The listing builds one solid part. Answer for the finished solid, in the listing's coordinates (mm). A direction names the side the tool comes from. Give positions to 0.01 mm unless a question says otherwise; leave off trailing zeros. Order: outer loops, then holes, each group sorted by start corner. A loop starts at its lowest first (then second) coordinate and runs counter-clockwise, first axis right, second up. Notation, with made-up numbers: (62.5, 57) -> (121.5, 57) arc R15 cw to (121.5, 69) -> close; hole circle Ø4 at (-27.5, -25). An arc over 180 degrees is marked (long way). Answer as a JSON object with one key per item and string values. Group by question number.
```python
from build123d import *

# Parameters (mm, degrees)
SKETCH1_R           = 0.75
SKETCH1_R_2         = 0.5
BOSS_EXTRUDE1_DEPTH = 2


with BuildPart() as part:
    # Sketch1 → Boss-Extrude1 (new body)
    with BuildSketch(Plane.XY):
        with BuildLine():
            Line((3.1, 16.98), (-3.1, 16.98))
            ThreePointArc((-3.1, 16.98), (-6.635533906, 15.515533906), (-8.1, 11.98))
            Line((-8.1, 11.98), (-8.1, 6))
            Line((-8.1, 6), (-4.1, 6))
            Line((-4.1, 6), (-4.1, 4))
            Line((-4.1, 4), (-8.1, 4))
            Line((-8.1, 4), (-8.1, 2))
            ThreePointArc((-8.1, 2), (-7.514213562, 0.585786438), (-6.1, 0))
            Line((-6.1, 0), (6.1, 0))
            ThreePointArc((6.1, 0), (7.514213562, 0.585786438), (8.1, 2))
            Line((8.1, 2), (8.1, 4))
            Line((8.1, 4), (4.1, 4))
            Line((4.1, 4), (4.1, 6))
            Line((4.1, 6), (8.1, 6))
            Line((8.1, 6), (8.1, 11.98))
            ThreePointArc((8.1, 11.98), (6.635533906, 15.515533906), (3.1, 16.98))
        make_face()
        with Locations((-5.35, 2)):
            Circle(SKETCH1_R, mode=Mode.SUBTRACT)
        with Locations((-5.1, 13.98)):
            Circle(SKETCH1_R_2, mode=Mode.SUBTRACT)
        with Locations((-2.1, 8.5)):
            Circle(SKETCH1_R, mode=Mode.SUBTRACT)
        with Locations((2.1, 8.5)):
            Circle(SKETCH1_R, mode=Mode.SUBTRACT)
        with Locations((5.1, 13.98)):
            Circle(SKETCH1_R_2, mode=Mode.SUBTRACT)
        with Locations((5.35, 2)):
            Circle(SKETCH1_R, mode=Mode.SUBTRACT)
    extrude(amount=BOSS_EXTRUDE1_DEPTH)


solid = part.part
```
(1) A cutting plane is placed at A-A (y = 8.5). Determine the outline of the cut face in (x, z), and give its area (3 significant figures).
(2) A cutting plane is placed at D-D (x = -5.35). Determine the outline of the cut face in (y, z), and give its area (3 significant figures).
(3) A cutting plane is placed at B-B (x = -2.1). Determine the outline of the cut face in (y, z).
(4) Which of the six approach directions +Z, -Z, +X, -X, +Y, -Y give full straight-line access (tool end or side, diameter ignored) to faces 4 (the cylindrical face through (7.5, 0.57, 0.99)), 5 (the flat face through (6, 4, 1)), 6 (the flat face through (-4.1, 5, 1))?
(5) A cutting plane is placed at C-C (z = 0.55). Determine the outline of the cut face in (x, y), and give its area (3 significant figures).
(6) For a pull along Y with two mould halves and no side action, classify faces 1 (the cylindrical face through (5.37, 14.4, 0.99)), 2 (the flat face through (8.1, 3, 1)), 3 (the cylindrical face through (6.67, 15.48, 0.99)) as +Y half, -Y half, draft (parallel to the pull), parting line (faces both ways), or undercut.
(7) Find the intervals of material crossed by line 1 along Y through (x, z) = (5.1, 0.9); line 2 along X through (y, z) = (1.5, 1.15); line 3 along X through (y, z) = (9, 1.35), in increasing order. Write a range as [from, to].
Check sheet entries:
{
 "1": {"outline": "(-8.1, 0) -> (-2.85, 0) -> (-2.85, 2) -> (-8.1, 2) -> close; (-1.35, 0) -> (1.35, 0) -> (1.35, 2) -> (-1.35, 2) -> close; (2.85, 0) -> (8.1, 0) -> (8.1, 2) -> (2.85, 2) -> close", "area": "26.4 mm2"},
 "2": {"outline": "(0, 0) -> (1.25, 0) -> (1.25, 2) -> (0, 2) -> close; (2.75, 0) -> (4, 0) -> (4, 2) -> (2.75, 2) -> close; (6, 0) -> (13.55, 0) -> (13.55, 2) -> (6, 2) -> close; (14.41, 0) -> (16.45, 0) -> (16.45, 2) -> (14.41, 2) -> close", "area": "24.2 mm2"},
 "3": {"outline": "(0, 0) -> (7.75, 0) -> (7.75, 2) -> (0, 2) -> close; (9.25, 0) -> (16.98, 0) -> (16.98, 2) -> (9.25, 2) -> close"},
 "4": {"face 4": "+Z, -Z, +X, -Y", "face 5": "+Z, -Z, +X", "face 6": "+Z, -Z, -X"},
 "5": {"outline": "(-8.1, 2) arc R2 ccw to (-6.1, 0) -> (6.1, 0) arc R2 ccw to (8.1, 2) -> (8.1, 4) -> (4.1, 4) -> (4.1, 6) -> (8.1, 6) -> (8.1, 11.98) arc R5 ccw to (3.1, 16.98) -> (-3.1, 16.98) arc R5 ccw to (-8.1, 11.98) -> (-8.1, 6) -> (-4.1, 6) -> (-4.1, 4) -> (-8.1, 4) -> close; hole circle Ø1.5 at (-5.35, 2); hole circle Ø1 at (-5.1, 13.98); hole circle Ø1.5 at (-2.1, 8.5); hole circle Ø1.5 at (2.1, 8.5); hole circle Ø1.5 at (5.35, 2); hole circle Ø1 at (5.1, 13.98)", "area": "238 mm2"},
 "6": {"face 1": "undercut", "face 2": "draft", "face 3": "+Y half"},
 "7": {"line 1": "y = [0, 1.29], [2.71, 4], [6, 13.48], [14.48, 16.56]", "line 2": "x = [-8.04, -5.91], [-4.79, 4.79], [5.91, 8.04]", "line 3": "x = [-8.1, -2.66], [-1.54, 1.54], [2.66, 8.1]"}
}
